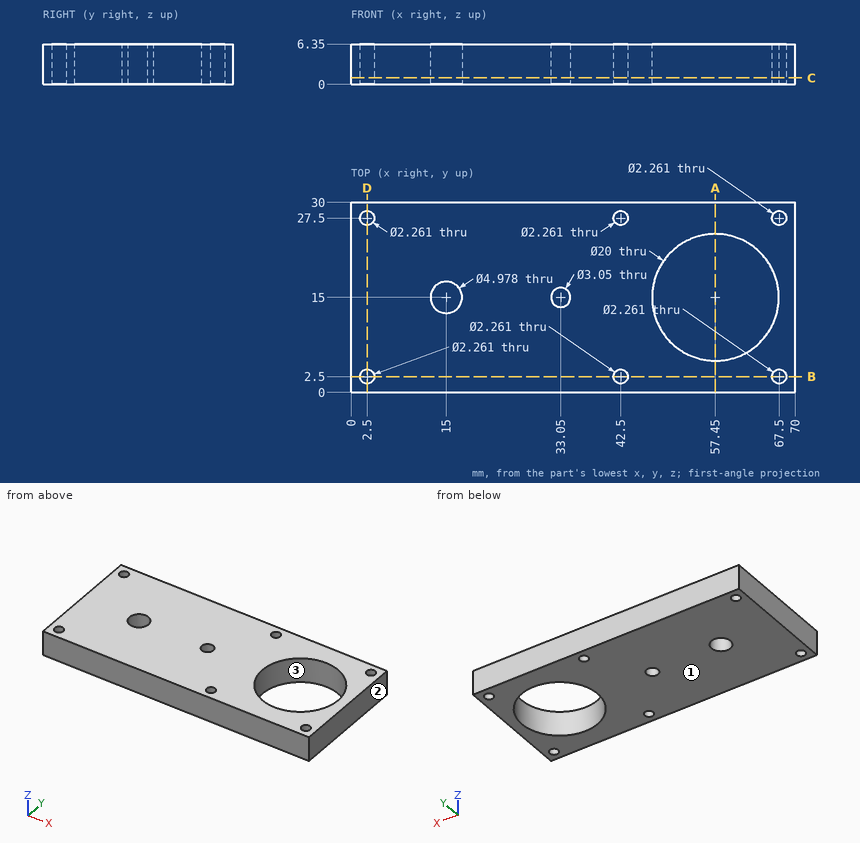
Geometry check sheet. Reference: drawing and pictorial views, mm from the part's lowest x, y, z. Round coordinates to 2 decimals unless told otherwise and drop trailing zeros. Loops run counter-clockwise (first coordinate to the right, second up) from the corner with the lowest first, then second, coordinate; pieces in that order, holes last. Notation, with made-up numbers: (-3.75, -12) -> (44.25, -12) arc R35 cw to (44.25, 27) -> close; hole circle Ø5 at (4.5, 52.25). An arc over 180 degrees is marked (long way). Use a Markdown table: item, result.
(1) Scan lines: probe 1 along Y at (x, z) = (42.5, 2.25); probe 2 along Y at (x, z) = (57.5, 3.25); probe 3 along X at (y, z) = (12.75, 1) (1 decimal). Record each from-to range of solid material in increasing order.
Calculated:
| item | result |
|---|---|
| probe 1 | 0 to 1.37, 3.63 to 26.37, 28.63 to 30 |
| probe 2 | 0 to 5, 25 to 30 |
| probe 3 | 0 to 13.9, 16.1 to 47.7, 67.2 to 70 |
(2) Sectioned sample at C-C (z = 1). Give the number of separate pieces and of enclosed holes in the cut face, then the cut area to 4 significant figures.
Calculated:
| item | result |
|---|---|
| separate pieces | 1 |
| enclosed holes | 9 |
| area | 1,735 mm² |
(3) Sectioned sample at D-D (x = 2.5). Enter the section's corners in (y, z).
Calculated:
| item | result |
|---|---|
| outline | (0, 0) -> (1.37, 0) -> (1.37, 6.35) -> (0, 6.35) -> close; (3.63, 0) -> (26.37, 0) -> (26.37, 6.35) -> (3.63, 6.35) -> close; (28.63, 0) -> (30, 0) -> (30, 6.35) -> (28.63, 6.35) -> close |
(4) Go/stop test with a flat-tipped pin: P1, Ø12, axis at x = 35.5, y = 13.5, coming from the -Z side. Record where the tip stops, or that it passes through.
Calculated:
| item | result |
|---|---|
| P1 | z = 0 |
(5) Mould release check, pull along X, two halves, no side actions. Record for the marked faces 1, 2 and 3: released by +X, released by -X, zero draft, split by the parting line, or undercut.
Calculated:
| item | result |
|---|---|
| face 1 | zero draft |
| face 2 | released by +X |
| face 3 | undercut |
(6) Sectioned sample at A-A (x = 57.45). Enter the section's corners in (y, z).
Calculated:
| item | result |
|---|---|
| outline | (0, 0) -> (5, 0) -> (5, 6.35) -> (0, 6.35) -> close; (25, 0) -> (30, 0) -> (30, 6.35) -> (25, 6.35) -> close |
(7) Sectioned sample at B-B (y = 2.5). Enter the section's corners in (x, z).
Calculated:
| item | result |
|---|---|
| outline | (0, 0) -> (1.37, 0) -> (1.37, 6.35) -> (0, 6.35) -> close; (3.63, 0) -> (41.37, 0) -> (41.37, 6.35) -> (3.63, 6.35) -> close; (43.63, 0) -> (66.37, 0) -> (66.37, 6.35) -> (43.63, 6.35) -> close; (68.63, 0) -> (70, 0) -> (70, 6.35) -> (68.63, 6.35) -> close |
